```python
from build123d import *

# Parameters (mm, degrees)
F0_R     = 3.175
F1_DEPTH = 38.1
F2_R     = 5.08
F2_R_2   = 3.175
F3_DEPTH = 6.35


# Not quite as in the source:
# - a pattern or mirror of a feature is missing from the dataset's text; its kind, count and spacing are read off the source's solid


with BuildPart() as f1:
    # F0 (on Right) → F1 (new body, symmetric)
    with BuildSketch(Plane.YZ):
        Circle(F0_R)
    extrude(amount=F1_DEPTH, both=True)

    # F2 (on face) → F3 (join)
    with BuildSketch(Plane.YZ.offset(38.1)):
        Circle(F2_R)
        Circle(F2_R_2, mode=Mode.SUBTRACT)
        Circle(F2_R_2)
    f3 = extrude(amount=F3_DEPTH)

    # F3_copies: F3 across plane
    add(f3.mirror(Plane(origin=(0, 0, 0), x_dir=(0, 0, -1), z_dir=(-1, 0, 0))))


solid = f1.part
```
The listing builds one solid part. Answer for the finished solid, in the listing's coordinates (mm). A direction names the side the tool comes from. Round coordinates to 2 decimals unless told otherwise and drop trailing zeros. Write each loop counter-clockwise with the first axis right and the second up, starting at its lowest first coordinate (ties: lowest second). Pieces come first, ordered by that corner, then holes. Notation, with made-up numbers: (66.5, 65) -> (90.5, 65) arc R24 ccw to (90.5, 95) -> close; hole circle Ø5 at (77, 29). An arc over 180 degrees is marked (long way). Use CSV: the item, a comma, the result in double quotes. Start each with the question number.
(1) Each of these flat-tipped pins is pushed along its axis until it touches: pin 1 (4 mm diameter, centred on x = -13, z = 2, fed in from -Y) (3 decimals); pin 2 (5 mm diameter, centred on x = -1.5, y = -1, fed in from +Z) (3 decimals); pin 3 (3 mm diameter, centred on x = 23.5, y = 3.5, fed in from -Z). Where does it stop, or does it pass through?
(2) Section C-C on z = 4 is taken. Give the vertices of the cut face in (x, y), then the cut area to 3 significant figures.
(3) Section D-D on x = -32 is taken. Give the vertices of the cut face in (y, z) (3 decimals).
(4) Consider L1, parallel to X at y = 3, z = -3.5; L2, parallel to Y at x = -35, z = -0.25. Determine where each line is inside the solid, lowest interval first. Write a range as from..to.
(5) Which of the six approach directions +Z, -Z, +X, -X, +Y, -Y give full straight-line access (tool end or side, diameter ignored) to faces 4 (the face through (-41.231, -0.661, 5.037)), 5 (the face through (-38.1, 3.3, -1.1))?
(6) Section A-A on y = 0 is taken. Give the vertices of the cut face in (x, z) (3 decimals).
(7) The mould has two halves that part along X. Classify faces 1 (the face through (0.53, -0.69, -3.1)), 2 (the face through (44.45, 0, 0)), 3 (the face through (41.231, -0.661, 5.037)): released by +X, released by -X, zero draft, split by the parting line, or undercut.
A:
1,pin 1,"stops at y = -3.175"
1,pin 2,"stops at z = 3.175"
1,pin 3,"stops at z = -2.47"
2,outline,"(-44.45, -3.13) -> (-38.1, -3.13) -> (-38.1, 3.13) -> (-44.45, 3.13) -> close; (38.1, -3.13) -> (44.45, -3.13) -> (44.45, 3.13) -> (38.1, 3.13) -> close"
2,area,"79.5 mm²"
3,outline,"circle Ø6.35 at (0, 0)"
4,L1,"x = -44.45..-38.1, 38.1..44.45"
4,L2,"y = -3.17..3.17"
5,face 4,"+X, -X"
5,face 5,"none"
6,outline,"(-44.45, -5.08) -> (-38.1, -5.08) -> (-38.1, -3.175) -> (38.1, -3.175) -> (38.1, -5.08) -> (44.45, -5.08) -> (44.45, 5.08) -> (38.1, 5.08) -> (38.1, 3.175) -> (-38.1, 3.175) -> (-38.1, 5.08) -> (-44.45, 5.08) -> close"
7,face 1,"undercut"
7,face 2,"released by +X"
7,face 3,"zero draft"
